from build123d import *

# Parameters (mm, degrees)
F1_DEPTH = 3.048
F3_DEPTH = 88.646


with BuildPart() as f1:
    # F0 (on Top) → F1 (new body)
    with BuildSketch(Plane.XY):
        Polygon((4.34401, -7.651717), (8.798587, -0.063836), (4.454577, 7.587881), (-4.34401, 7.651717), (-8.798587, 0.063836), (-4.454577, -7.587881), align=None)
    extrude(amount=F1_DEPTH)

    # F2 (on face) → F3 (cut)
    with BuildSketch(Plane.XY.offset(3.048)):
        Polygon((7.360816, -0.076723), (3.746852, 6.336292), (-3.613964, 6.413015), (-7.360816, 0.076723), (-3.746852, -6.336292), (3.613964, -6.413015), align=None)
    extrude(amount=-F3_DEPTH, mode=Mode.SUBTRACT)


solid = f1.part
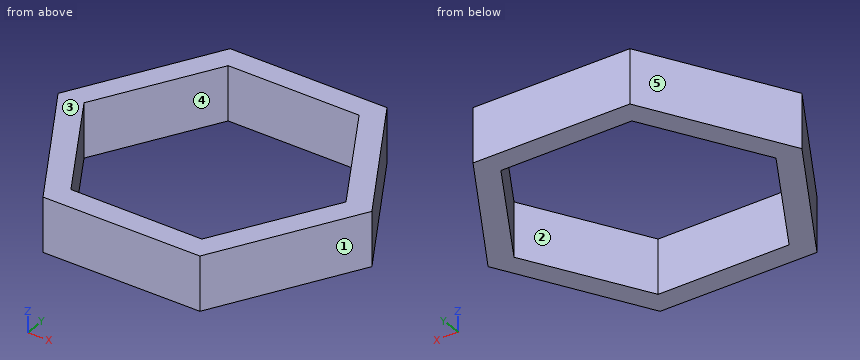
Design review of the part built by this model. Coordinates are the model's own, in mm. Face numbers are marked on the shaded views. A direction names the side the tool comes from. Coordinates: 2 decimals unless noted, no trailing zeros. Loops run counter-clockwise (first coordinate to the right, second up) from the corner with the lowest first, then second, coordinate; pieces in that order, holes last.
Item 1: Draft analysis for pull direction Y (two halves, no side actions). For the marked faces 1, 2 and 3, state which applies: pulls with the +Y half, pulls with the -Y half, needs draft (parallel to the pull), parting line crosses it, or undercut.
Completed:
face 1: pulls with the -Y half
face 2: undercut
face 3: needs draft
Item 2: Add section B-B (x = -4.75). Write out the cut boundary in (y, z).
Completed:
outline: (-7.07, 0) - (-4.56, 0) - (-4.56, 3.05) - (-7.07, 3.05) - close; (4.49, 0) - (6.96, 0) - (6.96, 3.05) - (4.49, 3.05) - close
Item 3: For the marked faces 4 and 5, list the 3-axis set-ups (+Z, -Z, +X, -X, +Y, -Y) from which the entire face can be reached by the end or side of a thin tool; tool diameter is ignored.
Completed:
face 4: +Z, -Z
face 5: +Z, -Z, -X, +Y
Item 4: Wall thickness on L1, parallel to X at y = -1.25, z = 2; L2, parallel to Y at x = 6, z = 1.25; L3, parallel to X at y = 3, z = 1: over which ranges is each line inside the solid? List them lowest first.
Completed:
L1: x = -8.05 to -6.61, 6.67 to 8.1
L2: y = -4.83 to -2.38, 2.34 to 4.87
L3: x = -7.07 to -5.63, 5.63 to 7.06
Item 5: Clearance check with flat-ended pins moving along their axes: pin 1 (6 mm diameter, centred on x = 6.5, y = -2, fed in from -Z); pin 2 (1.5 mm diameter, centred on x = 1.5, z = 2, fed in from -Y). State where each tip first meets the part, or that it passes through.
Completed:
pin 1: stops at z = 0
pin 2: stops at y = -7.64
Item 6: Add section C-C (y = 1.25). Write out the cut boundary in (x, z), and give its area (3 significant figures).
Completed:
outline: (-8.1, 0) - (-6.67, 0) - (-6.67, 3.05) - (-8.1, 3.05) - close; (6.61, 0) - (8.05, 0) - (8.05, 3.05) - (6.61, 3.05) - close
area: 8.76 mm2
Item 7: Add section A-A (z = 2.6). Write out the cut boundary in (x, y), and give its area (3 significant figures).
Completed:
outline: (-8.8, 0.06) - (-4.45, -7.59) - (4.34, -7.65) - (8.8, -0.06) - (4.45, 7.59) - (-4.34, 7.65) - close; hole (-7.36, 0.08) - (-3.75, -6.34) - (3.61, -6.41) - (7.36, -0.08) - (3.75, 6.34) - (-3.61, 6.41) - close
area: 60.4 mm2
